from build123d import *

# Parameters (mm, degrees)
SKETCH_2_R               = 2.5
CUT_EXTRUDE_1_DEPTH      = 10
CUT_EXTRUDE_START        = -10
CUT_EXTRUDE_3_DEPTH      = 10
SKETCH_5_R               = 1.5
EXTRUDE_1_DEPTH          = 20.1
PATTERN_CIRCULAR_8_COUNT = 9
SKETCH_6_R               = 108.516625274
CUT_EXTRUDE_4_DEPTH      = 2


with BuildPart() as part:
    # ｽｹｯﾁ1 → 回転1 (revolve)
    with BuildSketch(Plane.XY, mode=Mode.PRIVATE) as revolve_1_sk:
        Polygon((-15, -3.484577548), (-15, -0.484577548), (-28.5, -0.484577548), (-28.5, 1.515422452), (-46, 1.515422452), (-46, -0.484577548), (-45.9999, -3.484577548), (-46, -5.484577548), (-28.5, -5.484577548), (-28.5, -3.484577548), align=None)
    revolve(revolve_1_sk.sketch.rotate(Axis((0, 0, 0), (0, 1, 0)), 270), axis=Axis((0, 0, 0), (0, 1, 0)))

    # ｽｹｯﾁ2 → ｶｯﾄ - 押し出し1 (cut)
    with BuildSketch(Plane(origin=(0, -0.484577548, 0), x_dir=(1, 0, 0), z_dir=(0, 1, 0))):
        with Locations(Location((0, 23.75, 0), (0, 0, 270))):
            Circle(SKETCH_2_R)
        with Locations(Location((20.56810334, 11.875, 0), (0, 0, 270))):
            Circle(SKETCH_2_R)
        with Locations(Location((20.56810334, -11.875, 0), (0, 0, 270))):
            Circle(SKETCH_2_R)
        with Locations(Location((0, -23.75, 0), (0, 0, 270))):
            Circle(SKETCH_2_R)
        with Locations(Location((-20.56810334, -11.875, 0), (0, 0, 270))):
            Circle(SKETCH_2_R)
        with Locations(Location((-20.56810334, 11.875, 0), (0, 0, 270))):
            Circle(SKETCH_2_R)
    extrude(amount=-CUT_EXTRUDE_1_DEPTH, mode=Mode.SUBTRACT)

    # ｽｹｯﾁ3 → ｶｯﾄ - 押し出し3 (cut)
    with BuildSketch(Plane(origin=(0, 1.515422452, 0), x_dir=(1, 0, 0), z_dir=(0, 1, 0)).offset(CUT_EXTRUDE_START)):
        with BuildLine():
            Line((4.340576232, 33.259012282), (2.102472879, 45.951927139))
            ThreePointArc((2.102472879, 45.951927139), (-7.987816173, 45.301156639), (-17.692162956, 42.461598768))
            Line((-17.692162956, 42.461598768), (-15.454059603, 29.768683911))
            ThreePointArc((-15.454059603, 29.768683911), (-14.63159697, 28.477676178), (-13.137147742, 28.14636476))
            Line((-13.137147742, 28.14636476), (2.718257082, 30.942100421))
            ThreePointArc((2.718257082, 30.942100421), (4.009264815, 31.764563054), (4.340576232, 33.259012282))
        make_face()
        with BuildLine():
            Line((8.0284955, 30.005762114), (21.9715045, 21.955762114))
            ThreePointArc((21.9715045, 21.955762114), (23.489142591, 21.755961269), (24.703555308, 22.687812921))
            Line((24.703555308, 22.687812921), (31.147917072, 33.849774919))
            ThreePointArc((31.147917072, 33.849774919), (23, 39.837168574), (13.740806456, 43.899774919))
            Line((13.740806456, 43.899774919), (7.296444692, 32.737812921))
            ThreePointArc((7.296444692, 32.737812921), (7.096643847, 31.220174831), (8.0284955, 30.005762114))
        make_face()
        with BuildLine():
            ThreePointArc((45.618904696, 5.908936816), (43.225860556, 15.732926593), (38.744299816, 24.796758494))
            Line((38.744299816, 24.796758494), (26.632861425, 20.388555425))
            ThreePointArc((26.632861425, 20.388555425), (25.504286137, 19.354406707), (25.43751647, 17.825129897))
            Line((25.43751647, 17.825129897), (30.944040777, 2.696078702))
            ThreePointArc((30.944040777, 2.696078702), (31.978189495, 1.567503415), (33.507466306, 1.500733748))
            Line((33.507466306, 1.500733748), (45.618904696, 5.908936816))
        make_face()
        with BuildLine():
            ThreePointArc((38.744299816, -24.796758494), (43.225860556, -15.732926593), (45.618904696, -5.908936816))
            Line((45.618904696, -5.908936816), (33.507466306, -1.500733748))
            ThreePointArc((33.507466306, -1.500733748), (31.978189495, -1.567503415), (30.944040777, -2.696078702))
            Line((30.944040777, -2.696078702), (25.43751647, -17.825129897))
            ThreePointArc((25.43751647, -17.825129897), (25.504286137, -19.354406707), (26.632861425, -20.388555425))
            Line((26.632861425, -20.388555425), (38.744299816, -24.796758494))
        make_face()
        with BuildLine():
            ThreePointArc((13.740806456, -43.899774919), (23, -39.837168574), (31.147917072, -33.849774919))
            Line((31.147917072, -33.849774919), (24.703555308, -22.687812921))
            ThreePointArc((24.703555308, -22.687812921), (23.489142591, -21.755961269), (21.9715045, -21.955762114))
            Line((21.9715045, -21.955762114), (8.0284955, -30.005762114))
            ThreePointArc((8.0284955, -30.005762114), (7.096643847, -31.220174831), (7.296444692, -32.737812921))
            Line((7.296444692, -32.737812921), (13.740806456, -43.899774919))
        make_face()
        with BuildLine():
            ThreePointArc((-17.692162956, -42.461598768), (-7.987816173, -45.301156639), (2.102472879, -45.951927139))
            Line((2.102472879, -45.951927139), (4.340576232, -33.259012282))
            ThreePointArc((4.340576232, -33.259012282), (4.009264815, -31.764563054), (2.718257082, -30.942100421))
            Line((2.718257082, -30.942100421), (-13.137147742, -28.14636476))
            ThreePointArc((-13.137147742, -28.14636476), (-14.63159697, -28.477676178), (-15.454059603, -29.768683911))
            Line((-15.454059603, -29.768683911), (-17.692162956, -42.461598768))
        make_face()
        with BuildLine():
            Line((-30.973437657, -12.870456857), (-40.846772695, -21.155168645))
            ThreePointArc((-40.846772695, -21.155168645), (-35.238044383, -29.568230046), (-27.92674174, -36.552661952))
            Line((-27.92674174, -36.552661952), (-18.053406702, -28.267950163))
            ThreePointArc((-18.053406702, -28.267950163), (-17.346592526, -26.910172763), (-17.806893036, -25.450286058))
            Line((-17.806893036, -25.450286058), (-28.155773552, -13.116970523))
            ThreePointArc((-28.155773552, -13.116970523), (-29.513550952, -12.410156347), (-30.973437657, -12.870456857))
        make_face()
        with BuildLine():
            Line((-32, 10.05), (-44.888723528, 10.05))
            ThreePointArc((-44.888723528, 10.05), (-46, 0), (-44.888723528, -10.05))
            Line((-44.888723528, -10.05), (-32, -10.05))
            ThreePointArc((-32, -10.05), (-30.585786438, -9.464213562), (-30, -8.05))
            Line((-30, -8.05), (-30, 8.05))
            ThreePointArc((-30, 8.05), (-30.585786438, 9.464213562), (-32, 10.05))
        make_face()
        with BuildLine():
            Line((-18.053406702, 28.267950163), (-27.92674174, 36.552661952))
            ThreePointArc((-27.92674174, 36.552661952), (-35.238044383, 29.568230046), (-40.846772695, 21.155168645))
            Line((-40.846772695, 21.155168645), (-30.973437657, 12.870456857))
            ThreePointArc((-30.973437657, 12.870456857), (-29.513550952, 12.410156347), (-28.155773552, 13.116970523))
            Line((-28.155773552, 13.116970523), (-17.806893036, 25.450286058))
            ThreePointArc((-17.806893036, 25.450286058), (-17.346592526, 26.910172763), (-18.053406702, 28.267950163))
        make_face()
    extrude(amount=CUT_EXTRUDE_3_DEPTH, mode=Mode.SUBTRACT)

    # ｽｹｯﾁ5 → ﾎﾞｽ - 押し出し1 (add)
    with BuildSketch(Plane(origin=(-9.897317918, 0, 1.745164186), x_dir=(-0.1736481776669516, 0, -0.9848077530122044), z_dir=(0.9848077530122044, 0, -0.1736481776669516))):
        with Locations((40.55, -1.984577548)):
            Circle(SKETCH_5_R)
    extrude_1 = extrude(amount=EXTRUDE_1_DEPTH)

    # 円形ﾊﾟﾀｰﾝ8: ﾎﾞｽ - 押し出し1 ×9 about axis
    pattern_circular_8_axis = Axis((0, 0, 0), (0, -1, 0))
    for i in range(1, PATTERN_CIRCULAR_8_COUNT):
        add(extrude_1.rotate(pattern_circular_8_axis, i * 360 / PATTERN_CIRCULAR_8_COUNT))

    # ｽｹｯﾁ6 → ｶｯﾄ - 押し出し4 (cut)
    with BuildSketch(Plane.XZ.offset(5.484577548)):
        Circle(SKETCH_6_R)
    extrude(amount=-CUT_EXTRUDE_4_DEPTH, mode=Mode.SUBTRACT)


solid = part.part
The model under review builds one solid part; all positions refer to its coordinate system, in mm. A direction names the side the tool comes from. Round coordinates to 2 decimals unless told otherwise and drop trailing zeros. Loops run counter-clockwise (first coordinate to the right, second up) from the corner with the lowest first, then second, coordinate; pieces in that order, holes last. Notation, with made-up numbers: (45, 59.5) -> (61, 59.5) arc R27 cw to (61, 78.5) -> close; hole circle Ø5 at (56, 45). An arc over 180 degrees is marked (long way). One line per question, with ' | ' between items. Start each with the question number.
Item 1: For pin 1 (2.5 mm diameter, centred on x = -39.5, y = 0, fed in from -Z); pin 2 (1.5 mm diameter, centred on x = -39, y = -2, fed in from +Z); pin 3 (5 mm diameter, centred on x = -11, z = 32.5, fed in from +Y); pin 4 (6 mm diameter, centred on x = -26, z = -29, fed in from +Y), all flat-tipped, find the tip position at first contact; note any pin that passes through.
Item 2: Add section B-B, the plane x = 0. Count the separate pieces of the cut face and the enclosed holes in it, then the cut area to 3 significant figures.
Item 3: Wall thickness on line 1 along X through (y, z) = (0.6, 0); line 2 along Z through (x, y) = (11, -0.6); line 3 along X through (y, z) = (-1.9, -8.5): over which ranges is each line inside the solid? List them lowest first. Write a range as [from, to].
Item 4: Add section A-A, the plane z = 0. Write out the cut boundary in (x, y), then the cut area to 3 significant figures.
Item 5: Draft analysis for pull direction X (two halves, no side actions). For faces 1 (the face through (-23.05, -1.02, -19.2)), 2 (the face through (-43.254, -1.02, 15.655)), 3 (the face through (8.069, -1.02, -45.287)), state which applies: +X half, -X half, draft (parallel to the pull), parting line (faces both ways), or undercut.
Item 6: Machinability: for faces 4 (the face through (27.82, 0.53, 6.18)), 5 (the face through (-7.151, -1.534, 41.367)), 6 (the face through (14.9, -1.02, -26.04)), which of the approach directions +Z, -Z, +X, -X, +Y, -Y give a long, thin tool a straight path to every point of the face, cutting with its end or side? Answer none if there is none.
Return value:
1) pin 1: stops at z = -21.07 | pin 2: stops at z = 20.23 | pin 3: passes through | pin 4: stops at y = -0.48
2) separate pieces: 6 | enclosed holes: 0 | area: 85.0 mm2
3) line 1: x = [-30, -28.5], [28.5, 46] | line 2: z = [-44.67, -39.15], [-28.29, -10.2], [10.2, 28.29], [39.15, 44.67] | line 3: x = [-42.05, -39.05], [-30.05, -12.36], [12.36, 28.83], [38.46, 41.65]
4) outline: circle Ø3 at (-40.55, -1.98); (-30, -3.48) -> (-15, -3.48) -> (-15, -0.48) -> (-28.5, -0.48) -> (-28.5, 1.52) -> (-30, 1.52) -> close; (15, -3.48) -> (46, -3.48) -> (46, 1.52) -> (28.5, 1.52) -> (28.5, -0.48) -> (15, -0.48) -> close | area: 183 mm2
5) face 1: undercut | face 2: -X half | face 3: +X half
6) face 4: +Y | face 5: none | face 6: +Y, -Y
